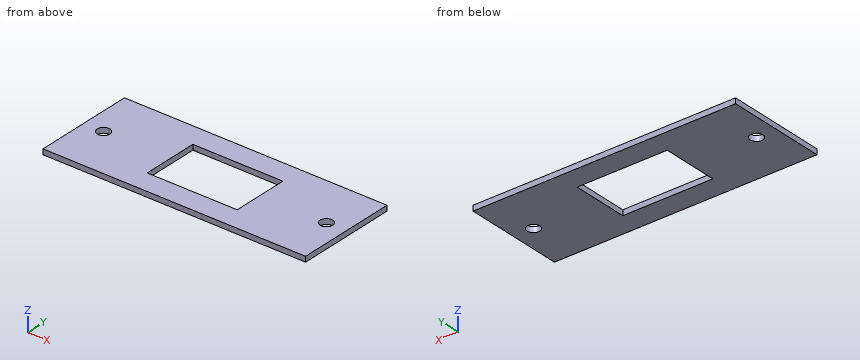
```python
from build123d import *

# Parameters (mm, degrees)
F0_W     = 99
F0_H     = 38
F0_W_2   = 33.95
F0_H_2   = 21.3
F1_DEPTH = 2
F2_R     = 2.38125
F3_DEPTH = 2.001


with BuildPart() as f1:
    # F0 (on Top) → F1 (new body)
    with BuildSketch(Plane.XY):
        with Locations((49.5, 19)):
            Rectangle(F0_W, F0_H)
        with Locations((49.5, 19)):
            Rectangle(F0_W_2, F0_H_2, mode=Mode.SUBTRACT)
    extrude(amount=F1_DEPTH)

    # F2 (on face) → F3 (cut, through all)
    with BuildSketch(Plane.XY.offset(2)):
        with Locations((7.5, 19)):
            Circle(F2_R)
        with Locations((91.5, 19)):
            Circle(F2_R)
    extrude(amount=-F3_DEPTH, mode=Mode.SUBTRACT)


solid = f1.part
```
Model file for the job. Use its own axes, mm. Give positions to 0.01 mm unless a question says otherwise; leave off trailing zeros. Loops run counter-clockwise (first coordinate to the right, second up) from the corner with the lowest first, then second, coordinate; pieces in that order, holes last. Notation, with made-up numbers: M 15,76 L 55,76 A12 ccw 55,90 Z; hole C 0.5,64.5 d3. An arc over 180 degrees is marked long. Use one line per item in the form item = value.
Item 1: Drill centre lines: L1, parallel to Y at x = 47.5, z = 0.1; L2, parallel to Y at x = 7.5, z = 1; L3, parallel to X at y = 22, z = 0.55 (3 decimals). Where is each one in solid material? Low to high.
Filled in:
L1 = 0 to 8.35, 29.65 to 38
L2 = 0 to 16.62, 21.38 to 38
L3 = 0 to 32.525, 66.475 to 99
Item 2: Slice it at A-A on y = 14. List the corners of the cut face in (x, z) (3 decimals).
Filled in:
outline = M 0,0 L 32.525,0 L 32.525,2 L 0,2 Z; M 66.475,0 L 99,0 L 99,2 L 66.475,2 Z
Item 3: Slice it at B-B on x = 7.5. List the corners of the cut face in (y, z), and give its area (3 significant figures).
Filled in:
outline = M 0,0 L 16.62,0 L 16.62,2 L 0,2 Z; M 21.38,0 L 38,0 L 38,2 L 21.38,2 Z
area = 66.5 mm^2
Item 4: Slice it at C-C on y = 19. List the corners of the cut face in (x, z) (3 decimals).
Filled in:
outline = M 0,0 L 5.119,0 L 5.119,2 L 0,2 Z; M 9.881,0 L 32.525,0 L 32.525,2 L 9.881,2 Z; M 66.475,0 L 89.119,0 L 89.119,2 L 66.475,2 Z; M 93.881,0 L 99,0 L 99,2 L 93.881,2 Z
Item 5: Flat gauge pins, fed straight in: pin 1 Ø5.5 at (x, y) = (91.5, 19) entering from +Z; pin 2 Ø4.5 at (x, y) = (7.5, 19) entering from +Z. Where does each tip first touch, or does it go through?
Filled in:
pin_1 = 2
pin_2 = through
Item 6: Slice it at D-D on z = 1.6. Give the number of separate pieces and of enclosed holes in the cut face, and give its area (3 significant figures).
Filled in:
separate_pieces = 1
enclosed_holes = 3
area = 3,000 mm^2
